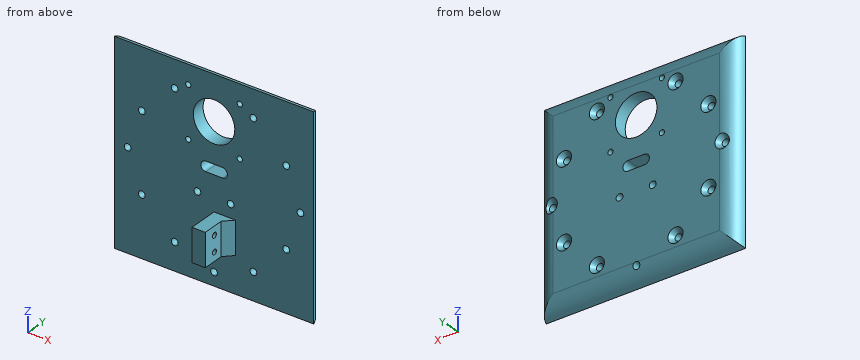
```python
from build123d import *

# Parameters (mm, degrees)
SKETCH1_W                                           = 120
SKETCH1_H                                           = 120
BOSS_EXTRUDE1_DEPTH                                 = 8
SKETCH2_R                                           = 12.5
SKETCH2_R_2                                         = 1.6
CUT_EXTRUDE1_DEPTH                                  = 86.229103011
SKETCH3_R                                           = 2.05
CUT_EXTRUDE2_DEPTH                                  = 86.229103011
CIRPATTERN1_COUNT                                   = 4
SKETCH4_R                                           = 2.05
CUT_EXTRUDE3_DEPTH                                  = 86.229103011
SKETCH5_R                                           = 2.05
CUT_EXTRUDE4_DEPTH                                  = 86.229103011
SKETCH6_W                                           = 8
SKETCH6_H                                           = 20
BOSS_EXTRUDE2_DEPTH                                 = 18
CHAMFER1_SIZE                                       = 5
SKETCH7_R                                           = 1.6
CUT_EXTRUDE5_DEPTH                                  = 93.455394651
CSK_FOR_M4_COUNTERSUNK_FLAT_HEAD_SCREW1_D           = 4.1
CSK_FOR_M4_COUNTERSUNK_FLAT_HEAD_SCREW1_DEPTH       = 7.999
CSK_FOR_M4_COUNTERSUNK_FLAT_HEAD_SCREW1_CSINK_D     = 9.1
CSK_FOR_M4_COUNTERSUNK_FLAT_HEAD_SCREW1_CSINK_ANGLE = 90
CSK_FOR_M4_COUNTERSUNK_FLAT_HEAD_SCREW1_TIP         = 1.231764269
FILLET1_R                                           = 10


with BuildPart() as part:
    # Sketch1 → Boss-Extrude1 (new body)
    with BuildSketch(Plane(origin=(0, 0, 0), x_dir=(1, 0, 0), z_dir=(0, 1, 0))):
        Rectangle(SKETCH1_W, SKETCH1_H)
    extrude(amount=BOSS_EXTRUDE1_DEPTH)

    # Sketch2 → Cut-Extrude1 (cut, through all)
    with BuildSketch(Plane(origin=(0, 8, 0), x_dir=(1, 0, 0), z_dir=(0, 1, 0))):
        with Locations(Location((0, -33, 0), (0, 0, 270))):
            Circle(SKETCH2_R)
        with Locations(Location((-15.5, -48.5, 0), (0, 0, 270))):
            Circle(SKETCH2_R_2)
        with Locations(Location((15.5, -48.5, 0), (0, 0, 270))):
            Circle(SKETCH2_R_2)
        with Locations(Location((15.5, -17.5, 0), (0, 0, 270))):
            Circle(SKETCH2_R_2)
        with Locations(Location((-15.5, -17.5, 0), (0, 0, 270))):
            Circle(SKETCH2_R_2)
    extrude(amount=-CUT_EXTRUDE1_DEPTH, mode=Mode.SUBTRACT)

    # Sketch3 → Cut-Extrude2 (cut, through all)
    with BuildSketch(Plane(origin=(0, 8, 0), x_dir=(1, 0, 0), z_dir=(0, 1, 0))):
        with Locations(Location((-43.487067043, -23.68807717, 0), (0, 0, 270))):
            Circle(SKETCH3_R)
        with Locations(Location((-23.68807717, -43.487067043, 0), (0, 0, 270))):
            Circle(SKETCH3_R)
    cut_extrude2 = extrude(amount=-CUT_EXTRUDE2_DEPTH, mode=Mode.SUBTRACT)

    # CirPattern1: Cut-Extrude2 ×4 about axis
    cirpattern1_axis = Axis((0, 0, 0), (0, 1, 0))
    for i in range(1, CIRPATTERN1_COUNT):
        add(cut_extrude2.rotate(cirpattern1_axis, i * 360 / CIRPATTERN1_COUNT), mode=Mode.SUBTRACT)

    # Sketch4 → Cut-Extrude3 (cut, through all)
    with BuildSketch(Plane(origin=(0, 8, 0), x_dir=(1, 0, 0), z_dir=(0, 1, 0))):
        with Locations(Location((-52, 0, 0), (0, 0, 270))):
            Circle(SKETCH4_R)
        with Locations(Location((52, 0, 0), (0, 0, 270))):
            Circle(SKETCH4_R)
        with Locations(Location((0, 52, 0), (0, 0, 270))):
            Circle(SKETCH4_R)
    extrude(amount=-CUT_EXTRUDE3_DEPTH, mode=Mode.SUBTRACT)

    # Sketch5 → Cut-Extrude4 (cut, through all)
    with BuildSketch(Plane(origin=(0, 8, 0), x_dir=(1, 0, 0), z_dir=(0, 1, 0))):
        with Locations(Location((-10, 10, 0), (0, 0, 270))):
            Circle(SKETCH5_R)
        with Locations(Location((10, 10, 0), (0, 0, 270))):
            Circle(SKETCH5_R)
        with BuildLine():
            Line((-5, -3), (5, -3))
            ThreePointArc((5, -3), (8, -6), (5, -9))
            Line((5, -9), (-5, -9))
            ThreePointArc((-5, -9), (-8, -6), (-5, -3))
        make_face()
    extrude(amount=-CUT_EXTRUDE4_DEPTH, mode=Mode.SUBTRACT)

    # Sketch6 → Boss-Extrude2 (add)
    with BuildSketch(Plane.XZ):
        with Locations((4, -28)):
            Rectangle(SKETCH6_W, SKETCH6_H)
    extrude(amount=BOSS_EXTRUDE2_DEPTH)

    # Chamfer1
    chamfer1_edges = [part.edges().sort_by_distance(p)[0] for p in [
        (8, 0, -28),
    ]]
    chamfer(chamfer1_edges, length=CHAMFER1_SIZE)

    # Sketch7 → Cut-Extrude5 (cut, through all)
    with BuildSketch(Plane(origin=(8, 0, 0), x_dir=(0, 0, -1), z_dir=(1, 0, 0))):
        with Locations((23.25, -10.5)):
            Circle(SKETCH7_R)
        with Locations((32.75, -10.5)):
            Circle(SKETCH7_R)
    extrude(amount=-CUT_EXTRUDE5_DEPTH, mode=Mode.SUBTRACT)

    # CSK for M4 Countersunk Flat Head Screw1
    with Locations(Plane(origin=(-52, 8, 0), x_dir=(0, 0, 1), z_dir=(0, 1, 0))):
        with Locations((0, 0), (23.68807717, 8.512932957), (43.487067043, 28.31192283), (43.487067043, 75.68807717), (23.68807717, 95.487067043), (0, 104), (-23.68807717, 95.487067043), (-43.487067043, 75.68807717), (-43.487067043, 28.31192283), (-23.68807717, 8.512932957)):
            CounterSinkHole(CSK_FOR_M4_COUNTERSUNK_FLAT_HEAD_SCREW1_D / 2, CSK_FOR_M4_COUNTERSUNK_FLAT_HEAD_SCREW1_CSINK_D / 2, depth=CSK_FOR_M4_COUNTERSUNK_FLAT_HEAD_SCREW1_DEPTH, counter_sink_angle=CSK_FOR_M4_COUNTERSUNK_FLAT_HEAD_SCREW1_CSINK_ANGLE)
            with Locations((0, 0, -(CSK_FOR_M4_COUNTERSUNK_FLAT_HEAD_SCREW1_DEPTH + CSK_FOR_M4_COUNTERSUNK_FLAT_HEAD_SCREW1_TIP / 2))):  # 118° drill point
                Cone(0, CSK_FOR_M4_COUNTERSUNK_FLAT_HEAD_SCREW1_D / 2, CSK_FOR_M4_COUNTERSUNK_FLAT_HEAD_SCREW1_TIP, mode=Mode.SUBTRACT)

    # Fillet1
    # the kernel refuses this fillet: 10 mm, written as the material it takes off along each edge
    with BuildSketch(Plane(origin=(-84.494897428, 8, -60), x_dir=(0, 0, 1), z_dir=(1, 0, 0)), Plane(origin=(60, 8, -84.494897428), x_dir=(-1, 0, 0), z_dir=(0, 0, 1)), Plane(origin=(-60, 8, 84.494897428), x_dir=(1, 0, 0), z_dir=(0, 0, -1)), Plane(origin=(84.494897428, 8, 60), x_dir=(0, 0, -1), z_dir=(-1, 0, 0))) as fillet1_piece_1:
        with BuildLine():
            CenterArc((9.797958971, 10), FILLET1_R, 191.536959033, 78.463040967)
            Line((0, 8), (0, 0))
            Line((0, 0), (9.797958971, 0))
        make_face()
    extrude(amount=168.989794856, mode=Mode.SUBTRACT)


solid = part.part
```
The listing builds one solid part. Answer for the finished solid, in the listing's coordinates (mm). Coordinates: 2 decimals unless noted, no trailing zeros. Write each loop counter-clockwise with the first axis right and the second up, starting at its lowest first coordinate (ties: lowest second). Pieces come first, ordered by that corner, then holes. Notation, with made-up numbers: (53, -27) - (93, -27) arc R18 cw to (93, 8) - close; hole circle Ø8 at (-18, 14.25). An arc over 180 degrees is marked (long way). Return JSON: item names as keys, results as strings. Group by question number.
1. A cutting plane is placed at A-A, the plane y = -10.5. Determine the outline of the cut face in (x, z), plus the area to 3 significant figures.
2. A cutting plane is placed at C-C, the plane z = 7.5. Determine the outline of the cut face in (x, y).
3. Given pin 1 (2 mm diameter, centred on x = 47.5, z = -45.5, fed in from -Y); pin 2 (4 mm diameter, centred on x = 5, y = -5, fed in from +Z); pin 3 (2.5 mm diameter, centred on x = 0.5, y = 4, fed in from -Z), each flat-ended and moving along its own axis, determine where each tip first touches the part or whether it passes through.
4. A cutting plane is placed at B-B, the plane x = -10. Determine the outline of the cut face in (y, z).
5. Straight lines are drawn through the part: L1, parallel to Y at x = 5.5, z = -32.75; L2, parallel to X at y = 1.1, z = 0; L3, parallel to Z at x = -16.5, y = 2.25. For each, find the intervals that lie inside material, in ascending order.
6. A cutting plane is placed at D-D, the plane x = -52. Determine the outline of the cut face in (y, z), plus the area to 3 significant figures.
Ans:
{
 "1": {"outline": "(0, -38) - (8, -38) - (8, -34.35) - (0, -34.35) - close; (0, -31.15) - (8, -31.15) - (8, -24.85) - (0, -24.85) - close; (0, -21.65) - (8, -21.65) - (8, -18) - (0, -18) - close", "area": "109 mm²"},
 "2": {"outline": "(-60, 0) - (-7.6, 0) - (-7.6, 8) - (-50.2, 8) arc R10 ccw to start; (7.6, 0) - (60, 0) arc R10 ccw to (50.2, 8) - (7.6, 8) - close"},
 "3": {"pin 1": "y = 0", "pin 2": "z = -18", "pin 3": "z = -59"},
 "4": {"outline": "(0, -60) arc R10 ccw to (8, -50.2) - (8, -12.05) - (0, -12.05) - close; (0, -7.95) - (8, -7.95) - (8, 25.5) - (0, 25.5) - close; (0, 40.5) - (8, 40.5) - (8, 50.2) arc R10 ccw to (0, 60) - close"},
 "5": {"L1": "-18 to -12.1, -8.9 to 8", "L2": "-59.71 to -54.05, -49.95 to 49.95, 54.05 to 59.71", "L3": "-59.25 to 16.25, 18.75 to 47.25, 49.75 to 59.25"},
 "6": {"outline": "(0, -60) arc R10 ccw to (7.84, -52) - (7.84, -4.39) - (5.5, -2.05) - (0, -2.05) - close; (0, 2.05) - (5.5, 2.05) - (7.84, 4.39) - (7.84, 52) arc R10 ccw to (0, 60) - close", "area": "866 mm²"}
}
